Part print with two shaded views. Sizes in mm from the minimum x, y, z corner. Give positions to 0.01 mm unless a question says otherwise; leave off trailing zeros. Order: outer loops, then holes, each group sorted by start corner. A loop starts at its lowest first (then second) coordinate and runs counter-clockwise, first axis right, second up. Notation, with made-up numbers: (-14.5, 67) - (-9.5, 67) arc R32 cw to (-9.5, 97) - close; hole circle Ø1 at (15, -3). An arc over 180 degrees is marked (long way). Return JSON: item names as keys, results as strings. Group by question number.
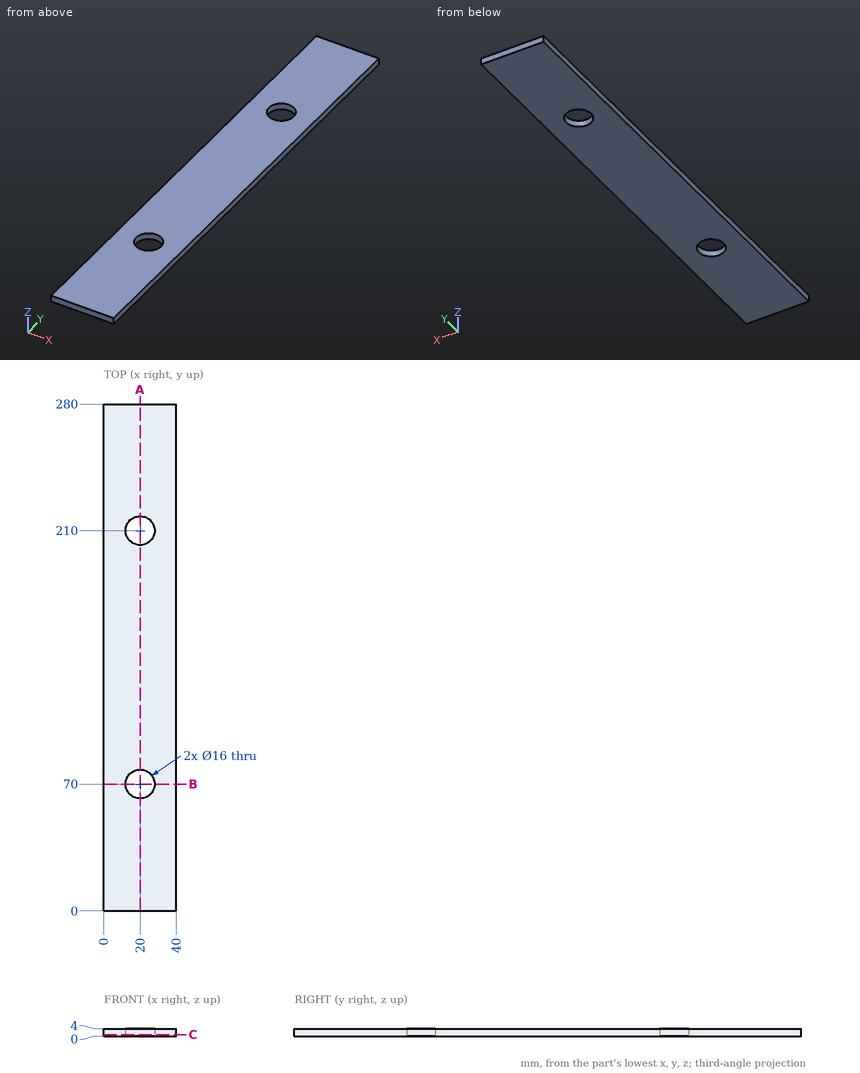
(1) Drill centre lines: L1, parallel to Y at x = 20, z = 2.05; L2, parallel to Y at x = 15.5, z = 3.05; L3, parallel to X at y = 213, z = 3.6. Where is each one in solid material? Low to high.
(2) Slice it at A-A (x = 20). Give the cut face in (y, z).
(3) Slice it at B-B (y = 70). Give the cut face in (x, z).
(4) Slice it at C-C (z = 0.7). Give the cut face in (x, y).
(5) Drop a flat-ended pin along its axis: pin 1 Ø14.5 at (x, y) = (20, 210) entering from +Z. Give the stop position or say it passes through.
Result set:
{
 "1": {"L1": "y = 0 to 62, 78 to 202, 218 to 280", "L2": "y = 0 to 63.39, 76.61 to 203.39, 216.61 to 280", "L3": "x = 0 to 12.58, 27.42 to 40"},
 "2": {"outline": "(0, 0) - (62, 0) - (62, 4) - (0, 4) - close; (78, 0) - (202, 0) - (202, 4) - (78, 4) - close; (218, 0) - (280, 0) - (280, 4) - (218, 4) - close"},
 "3": {"outline": "(0, 0) - (12, 0) - (12, 4) - (0, 4) - close; (28, 0) - (40, 0) - (40, 4) - (28, 4) - close"},
 "4": {"outline": "(0, 0) - (40, 0) - (40, 280) - (0, 280) - close; hole circle Ø16 at (20, 70); hole circle Ø16 at (20, 210)"},
 "5": {"pin 1": "passes through"}
}
